Input: part model. Units: mm. Frame: model coordinates. Coordinates: 2 decimals unless noted, no trailing zeros. Order: outer loops, then holes, each group sorted by start corner. A loop starts at its lowest first (then second) coordinate and runs counter-clockwise, first axis right, second up. Notation, with made-up numbers: (47, -13.5) -> (70, -13.5) arc R27 ccw to (70, 10.5) -> close; hole circle Ø6 at (-40, 10.5). An arc over 180 degrees is marked (long way). Write each question's results on one line, items separated by ' | '.
```python
from build123d import *

# Parameters (mm, degrees)
SKETCH2_W                = 3.4
SKETCH2_H                = 0.6
BOSS_EXTRUDE2_DEPTH      = 2.7
BOSS_EXTRUDE2_DEPTH_BACK = 5
SKETCH3_W                = 0.25
SKETCH3_H                = 0.1
CUT_EXTRUDE1_DEPTH       = 3
FILLET1_R                = 0.1


with BuildPart() as part:
    # Sketch2 → Boss-Extrude2 (new body, two sides)
    with BuildSketch(Plane.XY.offset(-3.5)) as boss_extrude2_sk:
        with Locations((0, 1.5)):
            Rectangle(SKETCH2_W, SKETCH2_H)
    extrude(amount=BOSS_EXTRUDE2_DEPTH)
    extrude(boss_extrude2_sk.sketch, amount=-BOSS_EXTRUDE2_DEPTH_BACK)

    # Sketch3 → Cut-Extrude1 (cut)
    with BuildSketch(Plane.XY.offset(-0.8)):
        with Locations((-1.3, 1.25)):
            Rectangle(SKETCH3_W, SKETCH3_H)
        with Locations((-0.65, 1.25)):
            Rectangle(SKETCH3_W, SKETCH3_H)
        with Locations((0, 1.25)):
            Rectangle(SKETCH3_W, SKETCH3_H)
        with Locations((0.65, 1.25)):
            Rectangle(SKETCH3_W, SKETCH3_H)
        with Locations((1.3, 1.25)):
            Rectangle(SKETCH3_W, SKETCH3_H)
    extrude(amount=-CUT_EXTRUDE1_DEPTH, mode=Mode.SUBTRACT)

    # Fillet1
    fillet1_edges = [part.edges().sort_by_distance(p)[0] for p in [
        (0, 1.8, -0.8),
        (1.7, 1.5, -0.8),
        (1.5625, 1.2, -0.8),
        (-1.5625, 1.2, -0.8),
        (-1.7, 1.5, -0.8),
        (0.975, 1.2, -0.8),
        (0.775, 1.25, -0.8),
        (0.65, 1.3, -0.8),
        (0.525, 1.25, -0.8),
        (0.325, 1.2, -0.8),
        (0.125, 1.25, -0.8),
        (0, 1.3, -0.8),
        (-0.125, 1.25, -0.8),
        (-0.325, 1.2, -0.8),
        (-0.525, 1.25, -0.8),
        (-0.65, 1.3, -0.8),
        (-0.775, 1.25, -0.8),
        (-0.975, 1.2, -0.8),
        (-1.175, 1.25, -0.8),
        (-1.3, 1.3, -0.8),
        (-1.425, 1.25, -0.8),
        (1.425, 1.25, -0.8),
        (1.3, 1.3, -0.8),
        (1.175, 1.25, -0.8),
    ]]
    fillet(fillet1_edges, radius=FILLET1_R)


solid = part.part
```
(1) Cut plane B-B, the plane x = 0.7. Return loops of the section in (y, z), plus the area to 3 significant figures.
Return value:
outline: (1.2, -8.5) -> (1.8, -8.5) -> (1.8, -0.9) arc R0.1 ccw to (1.7, -0.8) -> (1.4, -0.8) arc R0.1 ccw to (1.3, -0.9) -> (1.3, -3.8) -> (1.2, -3.8) -> close | area: 4.32 mm2
(2) Cut plane A-A, the plane z = -2.25. Return loops of the section in (x, y) (3 decimals), plus the area to 4 significant figures.
Return value:
outline: (-1.7, 1.2) -> (-1.425, 1.2) -> (-1.425, 1.3) -> (-1.175, 1.3) -> (-1.175, 1.2) -> (-0.775, 1.2) -> (-0.775, 1.3) -> (-0.525, 1.3) -> (-0.525, 1.2) -> (-0.125, 1.2) -> (-0.125, 1.3) -> (0.125, 1.3) -> (0.125, 1.2) -> (0.525, 1.2) -> (0.525, 1.3) -> (0.775, 1.3) -> (0.775, 1.2) -> (1.175, 1.2) -> (1.175, 1.3) -> (1.425, 1.3) -> (1.425, 1.2) -> (1.7, 1.2) -> (1.7, 1.8) -> (-1.7, 1.8) -> close | area: 1.915 mm2
(3) Line query: line 1 along X through (y, z) = (1.25, -3.25) (3 decimals). Output: solid intervals per line, ascending. Write a range as from..to.
Return value:
line 1: -1.7..-1.425, -1.175..-0.775, -0.525..-0.125, 0.125..0.525, 0.775..1.175, 1.425..1.7
